Verification items for the finished model (mm, model axes). A direction names the side the tool comes from. Round coordinates to 2 decimals unless told otherwise and drop trailing zeros. Write each loop counter-clockwise with the first axis right and the second up, starting at its lowest first coordinate (ties: lowest second). Pieces come first, ordered by that corner, then holes. Notation, with made-up numbers: M 1.25,2 L 7.25,2 A9 ccw 7.25,7 Z; hole C 82.5,-20 d7. An arc over 180 degrees is marked long. Write each question's results on one line, items separated by ' | '.
Autodesk Inventor part; units mm, degrees
ref_plane "YZ Plane" through (0, 0, 0) normal (1, 0, 0) x (0, 1, 0)
ref_plane "XZ Plane" through (0, 0, 0) normal (0, 1, 0) x (-1, 0, 0)
ref_plane "XY Plane" through (0, 0, 0) normal (0, 0, 1) x (1, 0, 0)
sketch "Skizze1" plane through (0, 0, 0) normal (0, 0, 1) x (1, 0, 0)
  line L0 (0, 0) -> (0, 50.2422)
  line L1 (0, 50.2422) -> (-42, 15)
  line L2 (-42, 15) -> (-42, 0)
  line L3 (-42, 0) -> (0, 0)
  line L4 (-6.5, 6.5) -> (-6.5, 36.3029)
  line L5 (-6.5, 36.3029) -> (-35.5, 11.969)
  line L6 (-35.5, 11.969) -> (-35.5, 6.5)
  line L7 (-35.5, 6.5) -> (-6.5, 6.5)
  dimension "d0" = 130
  dimension "d1" = 15
  dimension "d2" = 42
  dimension "d3" = 6.5
  dimension "d4" = 6.5
  dimension "d6" = 6.5
  dimension "d7" = 6.5
extrude "Extrusion1" add sketch "Skizze1" along normal blind 12
sketch "Skizze2" plane through (0, 0, 12) normal (0, 0, 1) x (1, 0, 0)
  line L0 (-3, 43.8087) -> (-3, 3)
  line L1 (-3, 3) -> (-39, 3)
  line L2 (-39, 3) -> (-39, 13.6011)
  line L3 (-39, 13.6011) -> (-3, 43.8087)
  line L4 (-42, 0) -> (0, 0)
  line L5 (-42, 15) -> (-42, 0)
  line L6 (0, 50.2422) -> (-42, 15)
  line L7 (0, 0) -> (0, 50.2422)
  dimension "d10" = 3
  dimension "d11" = 3
  dimension "d12" = 3
  dimension "d13" = 3
extrude "Extrusion2" cut sketch "Skizze2" against normal blind 9 contours L0 L1 L2 L3
sketch "Skizze3" plane through (-39, 3, 12) normal (0, 1, 0) x (1, 0, 0)
  line L0 (39, 12) -> (39, 0)
  line L1 (39, 0) -> (36, 0)
  line L2 (36, 0) -> (36, 9)
  line L3 (36, 9) -> (0, 9)
  line L4 (0, 9) -> (0, 0)
  line L5 (0, 0) -> (-3, 0)
  line L6 (-3, 0) -> (-3, 12)
  line L7 (-3, 12) -> (39, 12)
  line L8 (36, 0) -> (0, 0)
  line L9 (0, 4.5) -> (36, 4.5)
  point P0 (6, 4.5)
  point P1 (30, 4.5)
  dimension "d17" = 6
  dimension "d18" = 6
hole "Bohrung1" at (-33, 3, 7.5) at (-9, 3, 7.5) direction (0, -1, 0) diameter 2.7 depth 8 tip angle 118
fillet "Rundung2" radius 1 9 edges at (-6.5, 6.5, 1.5) (-3, 3, 7.5) (0, 50.2422, 6) (-6.5, 36.3029, 1.5) (-3, 43.8087, 7.5) (-39, 13.6011, 7.5) (-35.5, 11.969, 1.5) (-35.5, 6.5, 1.5) (-39, 3, 7.5)
sketch "Skizze4" plane through (-38.6428, 13.9008, 3) normal (0.6427876, -0.7660444, 0) x (0.7660444, 0.6427876, 0)
  line L0 (50.4446, -3) -> (-4.3825, -3)
  line L1 (-4.3825, -3) -> (-4.3825, 9)
  line L2 (-4.3825, 9) -> (0, 9)
  line L3 (0, 0) -> (0, 9)
  line L4 (0, 0) -> (44.3838, 0)
  line L5 (44.3838, 0) -> (44.3838, 9)
  line L6 (0, 9) -> (44.3838, 9)
  line L7 (50.4446, 9) -> (50.4446, -3)
  line L8 (44.3838, 9) -> (50.4446, 9)
  point P0 (20.6668, -3)
  point P1 (4, 5)
  point P2 (40, 6.5)
  dimension "d27" = 4
  dimension "d28" = 4
  dimension "d29" = 2.5
  dimension "d30" = 40
  dimension "d31" = 4.3838
hole "Bohrung2" at (-35.5786, 16.472, 8) at (-8.001, 39.6123, 9.5) direction (-0.6427876, 0.7660444, 0) diameter 2.5 depth 8 tip angle 118
sketch "Skizze5" plane through (-38.6428, 13.9008, 3) normal (0.6427876, -0.7660444, 0) x (0.7660444, 0.6427876, 0)
  circle A0 centre (40, 6.5) radius 1.25
  line L0 (41.25, 6.5) -> (41.25, 9)
  line L1 (50.8174, 9) -> (-1.8652, 9)
  line L2 (38.75, 9) -> (38.75, 6.5)
  point P0 (20.6668, -3)
extrude "Extrusion3" cut sketch "Skizze5" against normal blind 16.75 contours A0 L2 L1 L0
properties part number "oled_halterung_W162_rechts"
1) Sectioned sample at B-B, the plane z = 5.5. Record the cut outline in (x, y), and give its area (3 significant figures).
Calculated:
outline: M -42,0 L 0,0 L 0,48.1 A1 ccw -1.64,48.86 L -42,15 Z; hole M -39,4 A1 ccw -38,3 L -4,3 A1 ccw -3,4 L -3,41.66 A1 ccw -4.64,42.43 L -38.64,13.9 A1 ccw -39,13.13 Z | area: 445 mm²
2) Access from +Z, -Z, +X, -X, +Y, -Y to the whole of each face (thin tool, end or side, straight path). Record for faces 4 (the cylindrical face through (-37, 17, 7)), 5 (the flat face through (-21.881, 27.966, 7.563)), 6 (the flat face through (-35.5, 10, 1)).
Calculated:
face 4: none | face 5: +Z | face 6: +Z, -Z
3) Depth check by flat-ended pin: P1, Ø2.5, axis at x = -18.5, z = 8.5, coming from the +Y side; P2, Ø3, axis at x = -33, z = 7.5, coming from the +Y side; P3, Ø0.9, axis at x = -21, z = 1, coming from the +Y side. Enter the tip coordinate at first touch or a pass-through.
Calculated:
P1: stops at y = 35.77 | P2: stops at y = 23.81 | P3: stops at y = 33
4) Sectioned sample at C-C, the plane x = -17. Record the cut outline in (y, z), and give its area (3 significant figures).
Calculated:
outline: M 0,0 L 6.5,0 L 6.5,3 L 3,3 L 3,12 L 0,12 Z; M 27.49,0 L 35.98,0 L 35.98,12 L 32.06,12 L 32.06,3 L 27.49,3 Z | area: 107 mm²
5) Material ranges on line 1 (X direction, y = 2.15, z = 7.5); line 2 (Z direction, x = -9, y = 0.95); line 3 (X direction, y = 5.5, z = 4.5), recorded low to high. Write a range as [from, to].
Calculated:
line 1: x = [-42, -34.35], [-31.65, -10.35], [-7.65, 0] | line 2: z = [0, 6.15], [8.85, 12] | line 3: x = [-42, -39], [-3, 0]
6) Draft check along X on faces 1 (the flat face through (-21, 25, 0)), 2 (the cylindrical face through (-10.138, 1.479, 8.226)), 3 (the cylindrical face through (-0.563, 48.997, 6.084)). Enter one of: pulls with the +X half, pulls with the -X half, needs draft (parallel to the pull), parting line crosses it, or undercut.
Calculated:
face 1: needs draft | face 2: undercut | face 3: parting line crosses it
7) Sectioned sample at A-A, the plane y = 9.5. Record the cut outline in (x, z), and give its area (3 significant figures).
Calculated:
outline: M -42,0 L -35.5,0 L -35.5,3 L -39,3 L -39,12 L -42,12 Z; M -6.5,0 L 0,0 L 0,12 L -3,12 L -3,3 L -6.5,3 Z | area: 93.0 mm²
8) Sectioned sample at D-D, the plane x = -33. Record the cut outline in (y, z), and give its area (3 significant figures).
Calculated:
outline: M 0,0 L 6.5,0 L 6.5,3 L 3,3 L 3,6.15 L 0,6.15 Z; M 0,8.85 L 3,8.85 L 3,12 L 0,12 Z; M 14.07,0 L 22.55,0 L 22.55,12 L 18.64,12 L 18.64,3 L 14.07,3 Z | area: 99.1 mm²
